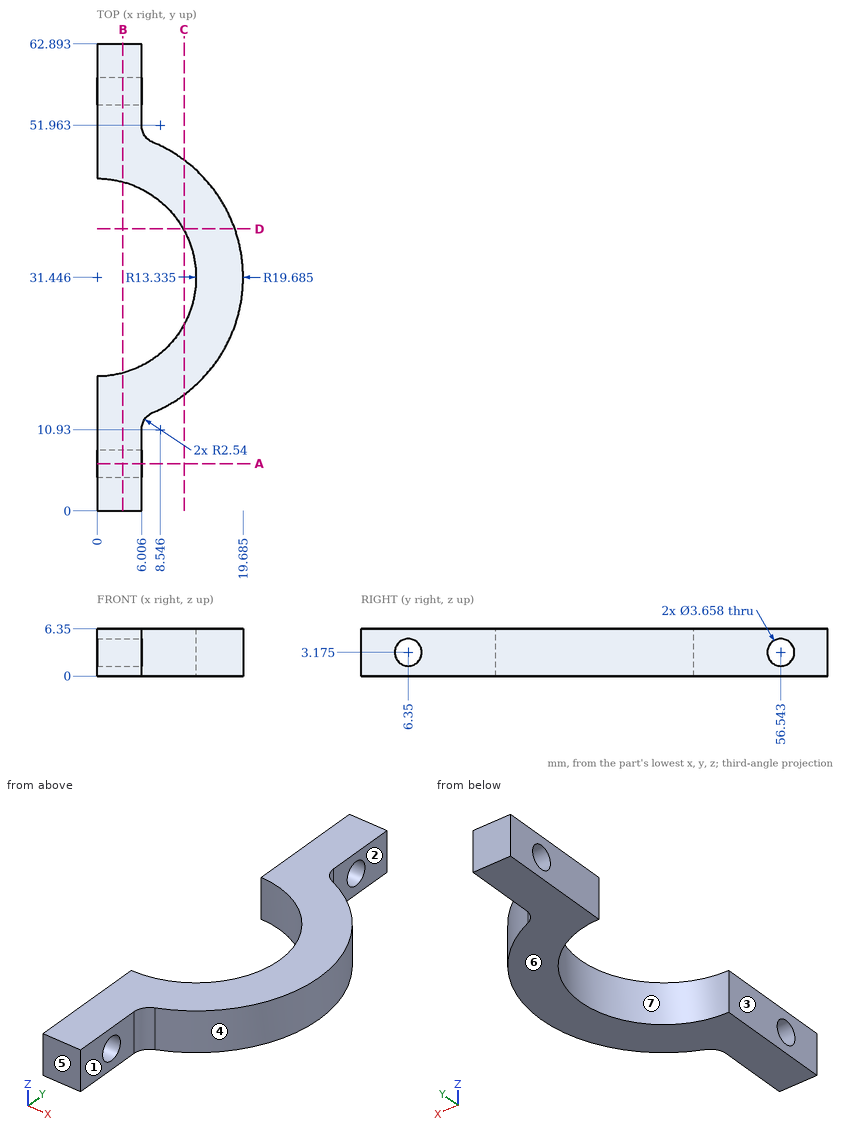
Study the drawing (mm; zero at the part's minimum x, y, z) and answer. A direction names the side the tool comes from. Give positions to 0.01 mm unless a question says otherwise; leave off trailing zeros. Loops run counter-clockwise (first coordinate to the right, second up) from the corner with the lowest first, then second, coordinate; pieces in that order, holes last. Notation, with made-up numbers: M -18,89.5 L 24,89.5 A19 cw 24,122.5 Z; hole C -16.75,-30 d9. An arc over 180 degrees is marked long. Answer as CSV lines item,"result".
Item 1: Which of the six approach directions +Z, -Z, +X, -X, +Y, -Y give full straight-line access (tool end or side, diameter ignored) to the marked faces 1, 2 and 3?
Values follow:
face 1,"+Z, -Z, +X, -Y"
face 2,"+Z, -Z, +X, +Y"
face 3,"+Z, -Z, -X, +Y, -Y"
Item 2: The part is cut by section D-D (y = 38). Give the vertices of the cut face in (x, z).
Values follow:
outline,"M 11.61,0 L 18.56,0 L 18.56,6.35 L 11.61,6.35 Z"
Item 3: The mould has two halves that part along Y. Classify the marked faces 4, 5, 6 and 7: released by +Y, released by -Y, zero draft, split by the parting line, or undercut.
Values follow:
face 4,"split by the parting line"
face 5,"released by -Y"
face 6,"zero draft"
face 7,"undercut"
Item 4: The part is cut by section A-A (y = 6.35). Give the vertices of the cut face in (x, z).
Values follow:
outline,"M 0,0 L 6.01,0 L 6.01,1.35 L 0,1.35 Z; M 0,5 L 6.01,5 L 6.01,6.35 L 0,6.35 Z"
Item 5: The part is cut by section B-B (x = 3.5). Give the number of separate pieces and of enclosed holes in the cut face, and give its area (3 significant figures).
Values follow:
separate pieces,"2"
enclosed holes,"2"
area,"215 mm^2"
Item 6: Straight lines are drawn through the part: line 1 along Y through (x, z) = (5.25, 1.5) (1 decimal); line 2 along Y through (x, z) = (5.75, 3.75) (1 decimal); line 3 along Z through (x, y) = (3.75, 6.35). For each, find the intervals that lie inside material, in ascending order. Write a range as [from, to].
Values follow:
line 1,"y = [0, 5.6], [7.1, 19.2], [43.7, 55.8], [57.3, 62.9]"
line 2,"y = [0, 4.6], [8.1, 19.4], [43.5, 54.8], [58.3, 62.9]"
line 3,"z = [0, 1.35], [5, 6.35]"
Item 7: The part is cut by section C-C (x = 11.75). Give the vertices of the cut face in (y, z).
Values follow:
outline,"M 15.65,0 L 25.14,0 L 25.14,6.35 L 15.65,6.35 Z; M 37.75,0 L 47.24,0 L 47.24,6.35 L 37.75,6.35 Z"
Item 8: Given pin 1 Ø3 at (y, z) = (3.5, 2) entering from +X; pin 2 Ø1 at (y, z) = (27.5, 5) entering from +X, each flat-ended and moving along its own axis, determine where each tip first touches the part or whether it passes through.
Values follow:
pin 1,"stops at x = 6.01"
pin 2,"stops at x = 19.38"
